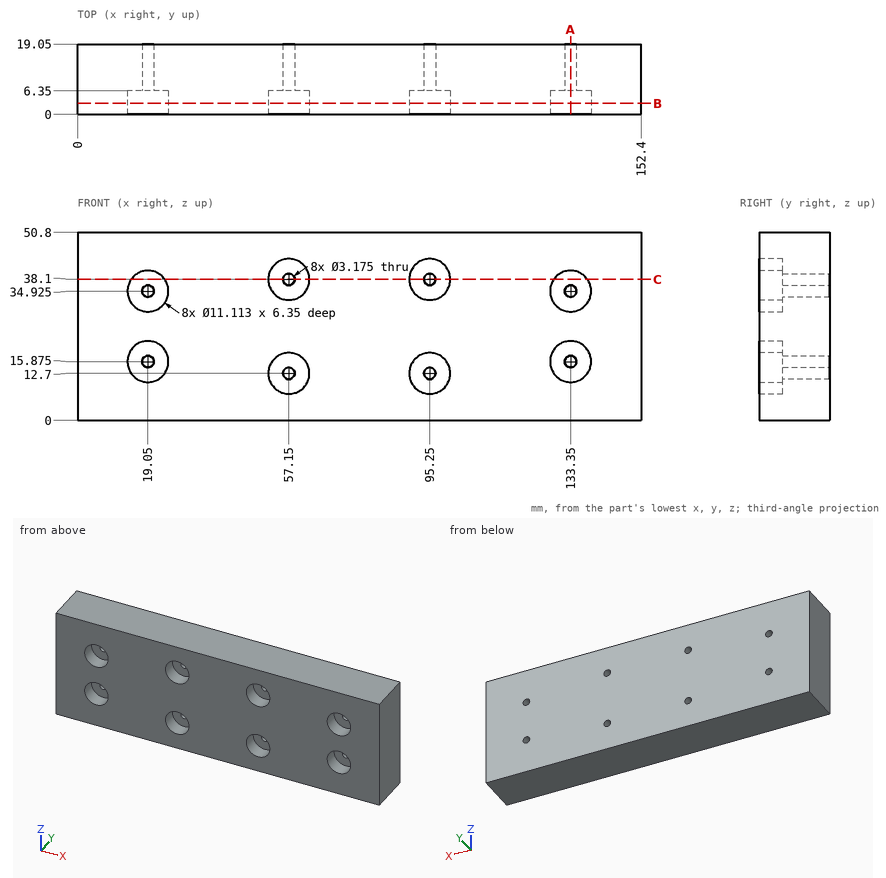
Job drawing, mm, ordinate dimensions from the low corner. One solid piece. Give positions to 0.01 mm unless a question says otherwise; leave off trailing zeros. Write each loop counter-clockwise with the first axis right and the second up, starting at its lowest first coordinate (ties: lowest second). Pieces come first, ordered by that corner, then holes. Notation, with made-up numbers: (-27, 44.25) -> (14, 44.25) arc R28 ccw to (14, 82.25) -> close; hole circle Ø7 at (36.25, -33). An arc over 180 degrees is marked (long way). Return JSON: item names as keys, results as strings.
Item 1: Drop a flat-ended pin along its axis: pin 1 (3.5 mm diameter, centred on x = 56.5, z = 13, fed in from -Y). Give the stop position or say it passes through.
Answer below:
{"pin 1": "stops at y = 6.35"}
Item 2: Band-saw the part on C-C (z = 38.1). List the corners of the cut face in (x, y).
Answer below:
{"outline": "(0, 0) -> (14.49, 0) -> (14.49, 6.35) -> (23.61, 6.35) -> (23.61, 0) -> (51.59, 0) -> (51.59, 6.35) -> (55.56, 6.35) -> (55.56, 19.05) -> (0, 19.05) -> close; (58.74, 6.35) -> (62.71, 6.35) -> (62.71, 0) -> (89.69, 0) -> (89.69, 6.35) -> (93.66, 6.35) -> (93.66, 19.05) -> (58.74, 19.05) -> close; (96.84, 6.35) -> (100.81, 6.35) -> (100.81, 0) -> (128.79, 0) -> (128.79, 6.35) -> (137.91, 6.35) -> (137.91, 0) -> (152.4, 0) -> (152.4, 19.05) -> (96.84, 19.05) -> close"}
Item 3: Drill centre lines: probe 1 along Z at (x, y) = (19.05, 12); probe 2 along Z at (x, y) = (95.25, 14.5); probe 3 along X at (y, z) = (4.25, 38.1) (1 decimal). Where is each one in solid material? Low to high.
Answer below:
{"probe 1": "z = 0 to 14.29, 17.46 to 33.34, 36.51 to 50.8", "probe 2": "z = 0 to 11.11, 14.29 to 36.51, 39.69 to 50.8", "probe 3": "x = 0 to 14.5, 23.6 to 51.6, 62.7 to 89.7, 100.8 to 128.8, 137.9 to 152.4"}
Item 4: Band-saw the part on A-A (x = 133.35). List the corners of the cut face in (y, z).
Answer below:
{"outline": "(0, 0) -> (19.05, 0) -> (19.05, 14.29) -> (6.35, 14.29) -> (6.35, 10.32) -> (0, 10.32) -> close; (0, 21.43) -> (6.35, 21.43) -> (6.35, 17.46) -> (19.05, 17.46) -> (19.05, 33.34) -> (6.35, 33.34) -> (6.35, 29.37) -> (0, 29.37) -> close; (0, 40.48) -> (6.35, 40.48) -> (6.35, 36.51) -> (19.05, 36.51) -> (19.05, 50.8) -> (0, 50.8) -> close"}
Item 5: Band-saw the part on B-B (y = 3). Give the number of separate pieces and of enclosed holes in the cut face, then the cut area to 3 significant figures.
Answer below:
{"separate pieces": "1", "enclosed holes": "8", "area": "6,970 mm2"}
